Autodesk Inventor part; units mm, degrees
ref_plane "YZ Plane" through (0, 0, 0) normal (1, 0, 0) x (0, 1, 0)
ref_plane "XZ Plane" through (0, 0, 0) normal (0, 1, 0) x (-1, 0, 0)
ref_plane "XY Plane" through (0, 0, 0) normal (0, 0, 1) x (1, 0, 0)
sketch "Sketch1" plane through (0, 0, 0) normal (0, 1, 0) x (-1, 0, 0)
  line L0 (0, 0) -> (9.5, 0)
  line L1 (9.5, 0) -> (9.5, -64)
  line L2 (9.5, -64) -> (0, -64)
  line L3 (0, -64) -> (0, 0)
  circle A0 centre (3.7, -11.5) radius 2.25
  circle A1 centre (3.7, -59.5) radius 2.25
  line L4 (3.7, -11.5) -> (3.7, -59.5) construction
  dimension "d1" = 9.5
  dimension "d2" = 64
  dimension "d3" = 4.5
  dimension "d4" = 48
  dimension "d6" = 3.7
  dimension "d17" = 4.5
extrude "Extrusion1" add sketch "Sketch1" along normal blind 12
sketch "Sketch2" plane through (-9.5, 0, 0) normal (0, 0, 1) x (1, 0, 0)
  line L0 (9.5, 12) -> (0, 12)
  line L1 (3, 12) -> (8.4, 12)
  line L2 (8.4, 12) -> (8.4, 10.8)
  line L3 (8.4, 10.8) -> (3, 10.8)
  line L4 (3, 10.8) -> (3, 12)
  line L5 (9.5, 0) -> (9.5, 12)
  line L6 (3.55, 0) -> (8.05, 0)
  line L7 (3.55, 12) -> (8.05, 12)
  line L8 (9.5, 0) -> (9.5, 12)
  line L9 (9.5, 0) -> (9.5, 12)
  line L10 (3.55, 12) -> (8.05, 12)
  line L11 (3.55, 12) -> (3.55, 0)
  line L12 (3.55, 12) -> (8.05, 12)
  line L13 (3.55, 0) -> (8.05, 0)
  line L14 (3.55, 12) -> (8.05, 12)
  line L15 (3.55, 0) -> (8.05, 0)
  line L16 (3.55, 12) -> (8.05, 12)
  line L17 (3.55, 0) -> (8.05, 0)
  dimension "d9" = 1.1
  dimension "d10" = 5.4
  dimension "d11" = 1.2
  dimension "d76" = 12
extrude "Extrusion2" cut sketch "Sketch2" against normal up to next
sketch "Sketch3" plane through (0, 0, 0) normal (0, -1, 0) x (1, 0, 0)
  circle A0 centre (-3.7, -11.5) radius 2.25
  circle A1 centre (-3.7, -11.5) radius 3.75
  circle A2 centre (-3.7, -59.5) radius 2.25
  circle A3 centre (-3.7, -59.5) radius 3.75
  point P0 (0, 0)
  dimension "d14" = 7.5
extrude "Extrusion3" cut sketch "Sketch3" against normal blind 3
fillet "Fillet1" radius 1 4 edges at (0, 1.5, -58.8897) (0, 1.5, -60.1103) (0, 1.5, -10.8897) (0, 1.5, -12.1103)
fillet "Fillet2" radius 4 2 edges at (-9.5, 6, -64) (-9.5, 6, 0)
sketch "Sketch28" plane through (0, 0, 0) normal (0, -1, 0) x (1, 0, 0)
  arc A0 (-1.5684, -56.4147) -> (0, -55.592) centre (-1, -55.592) ccw
  line L0 (0, -55.592) -> (0, -53)
  line L1 (0, -15.408) -> (0, -55.592)
  line L2 (-9.5, -60) -> (-9.5, -4)
  line L3 (0, -53) -> (-9.5, -53)
  line L4 (-9.5, -53) -> (-9.5, -31)
  line L5 (-9.5, -31) -> (0, -31)
  line L6 (0, -31) -> (0, -53)
  point P0 (0, 0)
  point P1 (0, -31)
  dimension "d107" = 2.592
  dimension "d108" = 22
extrude "Extrusion19" add sketch "Sketch28" along normal blind 10
sketch "Sketch29" plane through (0, -10, 0) normal (0, -1, 0) x (1, 0, 0)
  line L0 (-9.5, -53) -> (0, -53)
  line L1 (-9.5, -53) -> (38.5, -53)
  line L2 (38.5, -53) -> (38.5, -43)
  line L3 (38.5, -43) -> (-21.5, -43)
  line L4 (-21.5, -43) -> (-21.5, -53)
  line L5 (-21.5, -53) -> (-9.5, -53)
  point P0 (0, 0)
  dimension "d111" = 48
  dimension "d112" = 10
  dimension "d113" = 60
  dimension "d114" = 10
extrude "Extrusion20" add sketch "Sketch29" along normal blind 10
sketch "Sketch30" plane through (-21.5, -10, -53) normal (-1, 0, 0) x (0, 0, 1)
  arc A0 (10, -10) -> (10, -60) centre (41.225, -35) ccw
  point P0 (53, 10)
  dimension "d117" = 50
  dimension "d118" = 40
sketch "Sketch31" plane through (0, -20, 0) normal (0, -1, 0) x (1, 0, 0)
  line L0 (-21.5, -43) -> (-21.5, -53)
  line L1 (38.5, -43) -> (-21.5, -43)
  line L2 (-21.5, -53) -> (38.5, -53)
  line L3 (38.5, -53) -> (38.5, -43)
  line L4 (38.5, -43) -> (-21.5, -43)
  line L5 (-21.5, -43) -> (-21.5, -53)
  point P0 (0, 0)
sweep "Sweep1" add profiles "Sketch31" path "Sketch30"
properties part number "Back"
Part model, mm, in its own coordinate system. A direction names the side the tool comes from. Round coordinates to 2 decimals unless told otherwise and drop trailing zeros. Order: outer loops, then holes, each group sorted by start corner. A loop starts at its lowest first (then second) coordinate and runs counter-clockwise, first axis right, second up. Notation, with made-up numbers: M 41,-6 L 73,-6 A26 ccw 73,18 Z; hole C -35.75,15.25 d7. An arc over 180 degrees is marked long. Answer in a Markdown table with one row per item. Add a question column.
Q1. Mould opens along X. For faces 5 (the face through (38.5, -45, -52)), 6 (the face through (-16, -10, -48)), 7 (the face through (-4.91, 6.845, -13.397)), 8 (the face through (-8.359, 6.084, -1.203)) say: +X half, -X half, draft (parallel to the pull), parting line (faces both ways), or undercut.
Q2. Wall check: L1, parallel to Z at x = -3.7, y = 0.7; L2, parallel to Z at x = -3.7, y = 5.5; L3, parallel to Y at x = -8.5, z = -25. Give the ranges that are in metal, low to high. Write a range as from..to.
Q3. Cut at C-C on z = -46.5. Give the cut face in (x, y), and give its area (3 significant figures).
Q4. Cut at D-D on x = 28. Give the cut face in (y, z) (1 decimal).
Q5. Cut at A-A on z = -11.5. Give the cut face in (x, y), and give its area (3 significant figures).
Q6. Cut at B-B on y = 5.5. Give the cut face in (x, z).
Q7. 3-axis set-ups, long thin cutter, end or side, ignore diameter. For faces 1 (the face through (-1, 3, -59)), 2 (the face through (19, -10, -48)), 3 (the face through (-9.5, 3, -32)), 4 (the face through (8, -14, -53)): which of +Z, -Z, +X, -X, +Y, -Y reach the whole face in a straight line?
Q8. Pin check, flat tips, straight feed: pin 1 (0.6 mm diameter, centred on y = 11.5, z = -43, fed in from +X); pin 2 (8 mm diameter, centred on x = -4.5, z = -13.5, fed in from -Y); pin 3 (4 mm diameter, centred on x = 8, y = -40.5, fed in from -Z); pin 4 (6 mm diameter, centred on y = -14.5, z = -31.5, fed in from +X). Stop position of each tip, or through.
Established:
| question | item | result |
|---|---|---|
| 1 | face 5 | +X half |
| 1 | face 6 | draft |
| 1 | face 7 | undercut |
| 1 | face 8 | -X half |
| 2 | L1 | z = -64..-63.25, -55.75..-15.25, -7.75..0 |
| 2 | L2 | z = -64..-61.75, -57.25..-13.75, -9.25..0 |
| 2 | L3 | y = 0..12 |
| 3 | outline | M -21.5,-78.45 L 38.5,-78.45 L 38.5,-64.85 L -21.5,-64.85 Z; M -21.5,-25.15 L 38.5,-25.15 L 38.5,-10 L 0,-10 L 0,12 L -1.1,12 L -1.1,10.8 L -6.5,10.8 L -6.5,12 L -9.5,12 L -9.5,-10 L -21.5,-10 Z |
| 3 | area | 1,930 mm2 |
| 4 | outline | M -79.8,-45.2 A48.2 ccw -20,-53 L -10,-53 L -10,-43 L -20,-43 A40 cw -70,-43 Z |
| 5 | outline | M -9.5,0 L -7.45,0 L -7.45,3 L -5.95,3 L -5.95,10.8 L -6.5,10.8 L -6.5,12 L -9.5,12 Z; M -1.45,3 L 0,3 L 0,12 L -1.1,12 L -1.1,10.8 L -1.45,10.8 Z |
| 5 | area | 50.1 mm2 |
| 6 | outline | M -9.5,-60 A4 ccw -5.5,-64 L 0,-64 L 0,0 L -5.5,0 A4 ccw -9.5,-4 Z; hole C -3.7,-59.5 d4.5; hole C -3.7,-11.5 d4.5 |
| 7 | face 1 | none |
| 7 | face 2 | +Z, -Z, +X, +Y |
| 7 | face 3 | +Z, -Z, -X, +Y |
| 7 | face 4 | -Z, +X, -X |
| 8 | pin 1 | stops at x = 0 |
| 8 | pin 2 | stops at y = 0 |
| 8 | pin 3 | stops at z = -59.92 |
| 8 | pin 4 | passes through |
